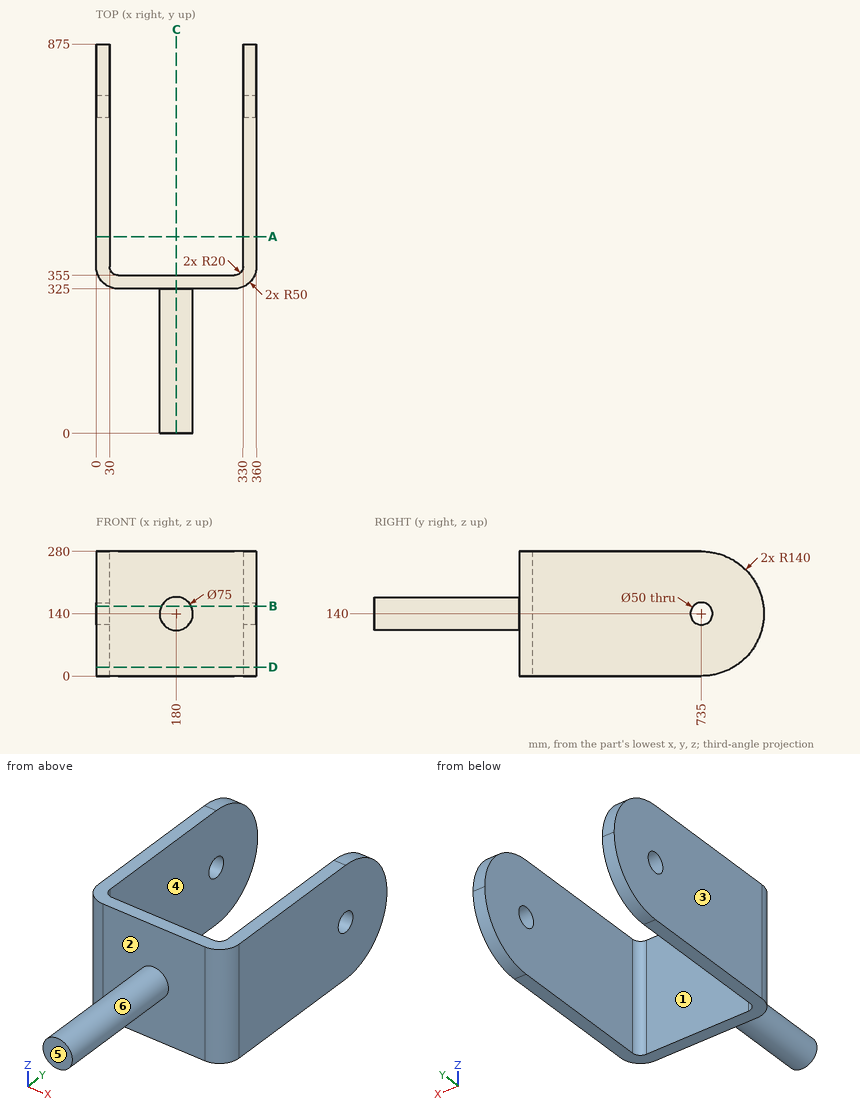
Print and shaded views of the part. All mm, measured from the part's lowest x, y and z. A direction names the side the tool comes from. Coordinates: 2 decimals unless noted, no trailing zeros. Loops run counter-clockwise (first coordinate to the right, second up) from the corner with the lowest first, then second, coordinate; pieces in that order, holes last. Notation, with made-up numbers: (87, 1) - (126, 1) arc R15 cw to (126, 18) - close; hole circle Ø4 at (1, 4.5). An arc over 180 degrees is marked (long way). Write item = value, one per line. Start each with the question number.
Item 1: Mould opens along X. For the marked faces 1, 2 and 3 say: released by +X, released by -X, zero draft, split by the parting line, or undercut.
Item 2: Cut at C-C, the plane x = 180. Give the cut face in (y, z), and give its area (3 significant figures).
Item 3: Cut at D-D, the plane z = 20. Give the cut face in (x, y), and give its area (3 significant figures).
Item 4: Wall check: L1, parallel to X at y = 385, z = 175; L2, parallel to Y at x = 143.5, z = 154.5; L3, parallel to Y at x = 338, z = 140 (1 decimal). Give the ranges that are in metal, low to high. Write a range as from..to.
Item 5: Cut at A-A, the plane y = 442. Give the cut face in (x, z).
Item 6: Flat gauge pins, fed straight in: pin 1 Ø1 at (x, z) = (138, 64) entering from -Y; pin 2 Ø1 at (y, z) = (170.5, 172.5) entering from -X. Where does each tip first touch, or does it go through?
Item 7: Cut at B-B, the plane z = 157. Give the cut face in (x, y).
Item 8: 3-axis set-ups, long thin cutter, end or side, ignore diameter. For the marked faces 4, 5 and 6: which of +Z, -Z, +X, -X, +Y, -Y reach the whole face in a straight line?
The answers:
q1.face_1 = undercut
q1.face_2 = zero draft
q1.face_3 = released by -X
q2.outline = (0, 102.5) - (325, 102.5) - (325, 0) - (355, 0) - (355, 280) - (325, 280) - (325, 177.5) - (0, 177.5) - close
q2.area = 32,800 mm2
q3.outline = (0, 375) arc R50 ccw to (50, 325) - (310, 325) arc R50 ccw to (360, 375) - (360, 807.11) - (330, 807.11) - (330, 375) arc R20 cw to (310, 355) - (50, 355) arc R20 cw to (30, 375) - (30, 807.11) - (0, 807.11) - close
q3.area = 37,000 mm2
q4.L1 = 0..30, 330..360
q4.L2 = 325..355
q4.L3 = 333.6..710, 760..875
q5.outline = (0, 0) - (30, 0) - (30, 280) - (0, 280) - close; (330, 0) - (360, 0) - (360, 280) - (330, 280) - close
q6.pin_1 = 325
q6.pin_2 = 160.45
q7.outline = (0, 375) arc R50 ccw to (50, 325) - (146.57, 325) - (146.57, 0) - (213.43, 0) - (213.43, 325) - (310, 325) arc R50 ccw to (360, 375) - (360, 716.67) - (330, 716.67) - (330, 375) arc R20 cw to (310, 355) - (50, 355) arc R20 cw to (30, 375) - (30, 716.67) - (0, 716.67) - close; (0, 753.33) - (30, 753.33) - (30, 873.96) - (0, 873.96) - close; (330, 753.33) - (360, 753.33) - (360, 873.96) - (330, 873.96) - close
q8.face_4 = +Z, -Z, +Y
q8.face_5 = +Z, -Z, +X, -X, -Y
q8.face_6 = -Y
